Design review of the part built by this model. Coordinates are the model's own, in mm. Face numbers are marked on the shaded views. A direction names the side the tool comes from. Coordinates: 2 decimals unless noted, no trailing zeros. Loops run counter-clockwise (first coordinate to the right, second up) from the corner with the lowest first, then second, coordinate; pieces in that order, holes last. Notation, with made-up numbers: (28, -20) - (71, -20) arc R15 cw to (71, 0) - close; hole circle Ø4 at (4.25, -4). An arc over 180 degrees is marked (long way). One line per question, with ' | ' between items.
from build123d import *

# Parameters (mm, degrees)
F0_R     = 2
F1_DEPTH = 10
F2_DEPTH = 30
F3_START = 27.5
F3_DEPTH = 2.5
F4_R     = 0.75


with BuildPart() as f1:
    # F0 (on Top) → F1 (new body)
    with BuildSketch(Plane.XY):
        Circle(F0_R)
    extrude(amount=F1_DEPTH)

    # F0 (on Top) → F2 (join)
    with BuildSketch(Plane.XY):
        Polygon((-3, 15.5884572681), (-9, 15.5884572681), (-18, 0), (-15, -5.1961524227), (-13.2792706909, -2.7386962898), (-9.0114159057, -10.1308376172), (-12, -10.3923048454), (-9, -15.5884572681), (9, -15.5884572681), (12, -10.3923048454), (9.0114159057, -10.1308376172), (13.2792706909, -2.7386962898), (15, -5.1961524227), (18, 0), (9, 15.5884572681), (3, 15.5884572681), (4.2678547852, 12.869533907), (-4.2678547852, 12.869533907), align=None)
        Circle(F0_R, mode=Mode.SUBTRACT)
    extrude(amount=F2_DEPTH)

    # F0 (on Top) → F3 (join)
    with BuildSketch(Plane.XY.offset(F3_START)):
        Polygon((3, 15.5884572681), (-3, 15.5884572681), (-4.2678547852, 12.869533907), (4.2678547852, 12.869533907), align=None)
        Polygon((-13.2792706909, -2.7386962898), (-15, -5.1961524227), (-12, -10.3923048454), (-9.0114159057, -10.1308376172), align=None)
        Polygon((12, -10.3923048454), (15, -5.1961524227), (13.2792706909, -2.7386962898), (9.0114159057, -10.1308376172), align=None)
    extrude(amount=F3_DEPTH)

    # F4
    f4_edges = [f1.edges().sort_by_distance(p)[0] for p in [
        (-2, 0, 30),
    ]]
    fillet(f4_edges, radius=F4_R)


solid = f1.part
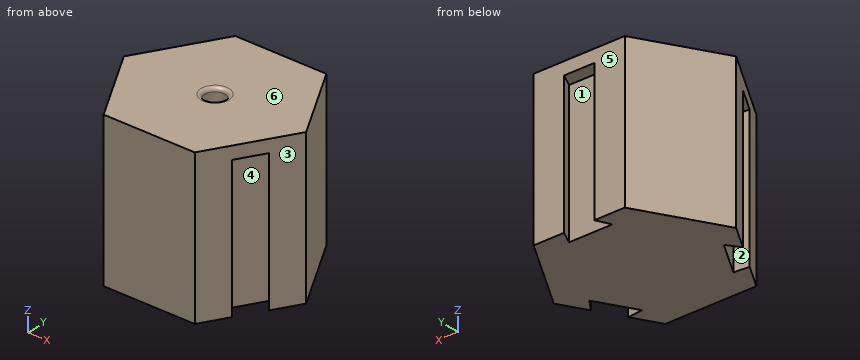
Q1. Take a section at A-A (z = 23). Give the boundary of the cut face in (x, y).
Returned:
outline: (-18, 0) - (-15, -5.2) - (-13.28, -2.74) - (-9.01, -10.13) - (-12, -10.39) - (-9, -15.59) - (9, -15.59) - (12, -10.39) - (9.01, -10.13) - (13.28, -2.74) - (15, -5.2) - (18, 0) - (9, 15.59) - (3, 15.59) - (4.27, 12.87) - (-4.27, 12.87) - (-3, 15.59) - (-9, 15.59) - close; hole circle Ø4 at (0, 0)
Q2. Draft analysis for pull direction Y (two halves, no side actions). For the marked faces 4, 5 and 6, state which applies: +Y half, -Y half, draft (parallel to the pull), parting line (faces both ways), or undercut.
Returned:
face 4: undercut | face 5: +Y half | face 6: draft
Q3. Take a section at C-C (z = 28.5). Give the boundary of the cut face in (x, y).
Returned:
outline: (-18, 0) - (-9, -15.59) - (9, -15.59) - (18, 0) - (9, 15.59) - (-9, 15.59) - close; hole circle Ø4 at (0, 0)
Q4. Take a section at D-D (y = 9.5). Give the boundary of the cut face in (x, z), plus the area to 3 significant figures.
Returned:
outline: (-12.52, 0) - (12.52, 0) - (12.52, 30) - (-12.52, 30) - close | area: 751 mm²
Q5. For pin 1 (4 mm diameter, centred on y = 3, z = 17, fed in from -X); pin 2 (2 mm diameter, centred on x = -1.5, y = 14.5, fed in from -Z); pin 3 (6 mm diameter, centred on x = -13.5, z = 8, fed in from -Y), all flat-tipped, find the tip position at first contact; note any pin that passes through.
Returned:
pin 1: stops at x = -17.42 | pin 2: stops at z = 27.5 | pin 3: stops at y = -12.99
Q6. To check wall thickness, follow line 1 along Y through (x, z) = (0, 24.25); line 2 along X through (y, z) = (-4.5, 3); line 3 along X through (y, z) = (-1, 13). State the ranges of each line that lie inside material, in increasing order.
Returned:
line 1: y = -15.59 to -2, 2 to 12.87 | line 2: x = -15.4 to -14.51, -12.26 to 12.26, 14.51 to 15.4 | line 3: x = -17.42 to -1.73, 1.73 to 17.42
Q7. Take a section at B-B (x = 0). Give the boundary of the cut face in (y, z).
Returned:
outline: (-15.59, 0) - (12.87, 0) - (12.87, 27.5) - (15.59, 27.5) - (15.59, 30) - (2.75, 30) arc R0.75 ccw to (2, 29.25) - (2, 10) - (-2, 10) - (-2, 29.25) arc R0.75 ccw to (-2.75, 30) - (-15.59, 30) - close
Q8. Tool access review of the marked faces 1, 2 and 3: name each direction out of +Z, -Z, +X, -X, +Y, -Y from which nothing blocks a thin tool from reaching the whole face with its end or side.
Returned:
face 1: -Z | face 2: -Z, -X | face 3: +Z, -Z, +X, -Y
